```python
from build123d import *

# Parameters (mm, degrees)
BOSS_EXTRUDE1_DEPTH = 20
CUT_EXTRUDE1_DEPTH  = 20
SKETCH3_W           = 20.5
SKETCH3_H           = 7
SKETCH3_H_2         = 7.25
CUT_EXTRUDE2_DEPTH  = 3


with BuildPart() as part:
    # Sketch1 → Boss-Extrude1 (new body)
    with BuildSketch(Plane(origin=(0, 0, 0), x_dir=(1, 0, 0), z_dir=(0, 1, 0))):
        with BuildLine():
            Line((0, 0), (50, 0))
            Line((50, 0), (50, 40.75))
            ThreePointArc((50, 40.75), (25, 65.75), (0, 40.75))
            Line((0, 40.75), (0, 0))
        make_face()
    extrude(amount=BOSS_EXTRUDE1_DEPTH)

    # Sketch2 → Cut-Extrude1 (cut)
    with BuildSketch(Plane(origin=(0, 20, 0), x_dir=(1, 0, 0), z_dir=(0, 1, 0))):
        Polygon((14.75, 8), (35.25, 8), (35.25, 48.75), (29, 48.75), (29, 53.75), (21, 53.75), (21, 48.75), (14.75, 48.75), align=None)
    extrude(amount=-CUT_EXTRUDE1_DEPTH, mode=Mode.SUBTRACT)

    # Sketch3 → Cut-Extrude2 (cut)
    with BuildSketch(Plane(origin=(0, 20, 0), x_dir=(1, 0, 0), z_dir=(0, 1, 0))):
        with Locations((25, 52.25)):
            Rectangle(SKETCH3_W, SKETCH3_H)
        with Locations((25, 4.375)):
            Rectangle(SKETCH3_W, SKETCH3_H_2)
    extrude(amount=-CUT_EXTRUDE2_DEPTH, mode=Mode.SUBTRACT)


solid = part.part
```
Build history of the part. All positions in model axes, mm. A direction names the side the tool comes from. Give positions to 0.01 mm unless a question says otherwise; leave off trailing zeros. Loops run counter-clockwise (first coordinate to the right, second up) from the corner with the lowest first, then second, coordinate; pieces in that order, holes last.
Item 1: Which spindle directions (+Z, -Z, +X, -X, +Y, -Y) get a long thin tool onto all of the face, cutting with end or side? Do faces 4 (the face through (36, 20, -33)), 5 (the face through (25, 9, -53.75)), 6 (the face through (25, 19, -55.75)). Say none if no direction does.
Answers follow:
face 4: +Z, -Z, +X, -X, +Y
face 5: +Y, -Y
face 6: +Y
Item 2: Slice it at A-A, the plane z = -23. List the corners of the cut face in (x, y).
Answers follow:
outline: (0, 0) - (14.75, 0) - (14.75, 20) - (0, 20) - close; (35.25, 0) - (50, 0) - (50, 20) - (35.25, 20) - close
Item 3: Slice it at B-B, the plane x = 25. List the corners of the cut face in (y, z), and give its area (3 significant figures).
Answers follow:
outline: (0, -65.75) - (20, -65.75) - (20, -55.75) - (17, -55.75) - (17, -53.75) - (0, -53.75) - close; (0, -8) - (17, -8) - (17, -0.75) - (20, -0.75) - (20, 0) - (0, 0) - close
area: 372 mm2
Item 4: Slice it at D-D, the plane x = 20. List the corners of the cut face in (y, z).
Answers follow:
outline: (0, -65.24) - (20, -65.24) - (20, -55.75) - (17, -55.75) - (17, -48.75) - (0, -48.75) - close; (0, -8) - (17, -8) - (17, -0.75) - (20, -0.75) - (20, 0) - (0, 0) - close
Item 5: Pull direction X, two halves, no side cores. Call faces 1 (the face through (0, 10, -21)), 2 (the face through (25, 9, -8)), 3 (the face through (25, 10, 0)): released by +X, released by -X, zero draft, split by the parting line, or undercut.
Answers follow:
face 1: released by -X
face 2: undercut
face 3: zero draft
Item 6: Slice it at C-C, the plane y = 9. List the corners of the cut face in (x, z), and give its area (3 significant figures).
Answers follow:
outline: (0, -40.75) arc R25 ccw to (50, -40.75) - (50, 0) - (0, 0) - close; hole (14.75, -48.75) - (21, -48.75) - (21, -53.75) - (29, -53.75) - (29, -48.75) - (35.25, -48.75) - (35.25, -8) - (14.75, -8) - close
area: 2,140 mm2
Item 7: Flat gauge pins, fed straight in: pin 1 (8 mm diameter, centred on x = 44.5, y = 18, fed in from +Z); pin 2 (4 mm diameter, centred on y = 9.5, z = -50.5, fed in from -X); pin 3 (6 mm diameter, centred on x = 26.5, z = -4, fed in from +Y); pin 4 (12 mm diameter, centred on x = 23, z = -24, fed in from +Y). Where does each tip first touch, or does it go through?
Answers follow:
pin 1: stops at z = 0
pin 2: stops at x = 1.23
pin 3: stops at y = 17
pin 4: passes through
Item 8: Drill centre lines: line 1 (X direction, y = 17.5, z = -13); line 2 (Z direction, x = 35, y = 9); line 3 (X direction, y = 15, z = -48). Where is each one in solid material? Low to high.
Answers follow:
line 1: x = 0 to 14.75, 35.25 to 50
line 2: z = -63.66 to -48.75, -8 to 0
line 3: x = 1.07 to 14.75, 35.25 to 48.93
